```python
from build123d import *

# Parameters (mm, degrees)
SKETCH_R        = 12
SKETCH_R_2      = 1.75
PAD_DEPTH       = 5
PAD001_DEPTH    = 45
PAD002_DEPTH    = 19
POCKET_DEPTH    = 1
SKETCH004_R     = 4.15
POCKET001_DEPTH = 48.001
SKETCH005_R     = 2.6
POCKET002_DEPTH = 42.301
SKETCH006_R     = 2.6
POCKET003_DEPTH = 5
SKETCH008_R     = 1.75
POCKET004_DEPTH = 20.801
SKETCH009_R     = 3.2
POCKET005_DEPTH = 3
POCKET006_DEPTH = 4
SKETCH011_W     = 1
SKETCH011_H     = 8
POCKET007_DEPTH = 18.99
FILLET_R        = 1
FILLET001_R     = 0.5
CHAMFER_SIZE    = 0.49


with BuildPart() as part:
    # Sketch → Pad (new body)
    with BuildSketch(Plane.XY):
        Polygon((0, 0), (-24, 0), (-24, 5), (-15.5, 5), (-15.5, 25), (-24, 25), (-24, 38.3), (-20, 42.3), (26, 42.3), (30, 38.3), (30, 4), (5, -24), (0, -24), align=None)
        with Locations((8.85, 21.15)):
            Circle(SKETCH_R, mode=Mode.SUBTRACT)
        with Locations((-6.65, 36.65)):
            Circle(SKETCH_R_2, mode=Mode.SUBTRACT)
        with Locations((24.35, 36.65)):
            Circle(SKETCH_R_2, mode=Mode.SUBTRACT)
        with Locations((24.35, 5.65)):
            Circle(SKETCH_R_2, mode=Mode.SUBTRACT)
    extrude(amount=PAD_DEPTH)

    # Sketch001 (on Face19 of Pad) → Pad001 (join)
    with BuildSketch(Plane.XY.offset(5)):
        Polygon((0, 0), (-24, 0), (-24, 5), (5, 5), (5, -24), (0, -24), align=None)
    extrude(amount=PAD001_DEPTH)

    # Sketch002 (on Face21 of Pad001) → Pad002 (join)
    with BuildSketch(Plane(origin=(0, 5, 0), x_dir=(-1, 0, 0), z_dir=(0, 1, 0))):
        Polygon((24, 0), (24, 18), (18, 24), (9.2, 24), (3.2, 18), (3.2, 5), (16.5, 5), (16.5, 0), align=None)
    extrude(amount=PAD002_DEPTH)

    # Sketch003 (on Face30 of Pad002) → Pocket (cut)
    with BuildSketch(Plane(origin=(0, 5, 0), x_dir=(-1, 0, 0), z_dir=(0, 1, 0))):
        Polygon((15.5, 0), (15.5, 18), (19.75, 22.25), (24, 18), (24, 0), align=None)
    extrude(amount=POCKET_DEPTH, mode=Mode.SUBTRACT)

    # Sketch004 (on Face37 of Pocket) → Pocket001 (cut, through all)
    with BuildSketch(Plane(origin=(0, 24, 0), x_dir=(-1, 0, 0), z_dir=(0, 1, 0))):
        with Locations((13.6, 15.5)):
            Circle(SKETCH004_R)
    extrude(amount=-POCKET001_DEPTH, mode=Mode.SUBTRACT)

    # Sketch005 (on Face4 of Pocket001) → Pocket002 (cut, through all)
    with BuildSketch(Plane.XZ):
        with Locations((-15, 35)):
            Circle(SKETCH005_R)
    extrude(amount=-POCKET002_DEPTH, mode=Mode.SUBTRACT)

    # Sketch006 (on Face7 of Pocket002) → Pocket003 (cut)
    with BuildSketch(Plane(origin=(0, 0, 0), x_dir=(0, -1, 0), z_dir=(-1, 0, 0))):
        with Locations((15, 40)):
            Circle(SKETCH006_R)
        with Locations((15, 15)):
            Circle(SKETCH006_R)
    extrude(amount=-POCKET003_DEPTH, mode=Mode.SUBTRACT)

    # Sketch008 (on Face41 of Pocket003) → Pocket004 (cut, through all)
    with BuildSketch(Plane.YZ.offset(-3.2)):
        with Locations((15, 8.5)):
            Circle(SKETCH008_R)
    extrude(amount=-POCKET004_DEPTH, mode=Mode.SUBTRACT)

    # Sketch009 (on Face41 of Pocket004) → Pocket005 (cut)
    with BuildSketch(Plane.YZ.offset(-3.2)):
        with Locations((15, 8.5)):
            Circle(SKETCH009_R)
    extrude(amount=-POCKET005_DEPTH, mode=Mode.SUBTRACT)

    # Sketch010 (on Face43 of Pocket005) → Pocket006 (cut)
    with BuildSketch(Plane(origin=(-24, 0, 0), x_dir=(0, -1, 0), z_dir=(-1, 0, 0))):
        Polygon((-12.1, 6.825684), (-12.1, 10.174316), (-15, 11.848632), (-17.9, 10.174316), (-17.9, 6.825684), (-15, 5.151368), align=None)
    extrude(amount=-POCKET006_DEPTH, mode=Mode.SUBTRACT)

    # Sketch011 (on Face36 of Pocket006) → Pocket007 (cut)
    with BuildSketch(Plane(origin=(0, 24, 0), x_dir=(-1, 0, 0), z_dir=(0, 1, 0))):
        with Locations((16, 9)):
            Rectangle(SKETCH011_W, SKETCH011_H)
    extrude(amount=-POCKET007_DEPTH, mode=Mode.SUBTRACT)

    # Fillet
    fillet_edges = [part.edges().sort_by_distance(p)[0] for p in [
        (5, 5, 27.5),
        (-3.2, 24, 11.5),
        (-6.2, 24, 21),
        (-13.6, 24, 24),
        (-21, 24, 21),
        (-24, 24, 9),
        (30, 4, 2.5),
        (-24, 6, 9),
        (-21.875, 6, 20.125),
        (-19.75, 5.5, 22.25),
        (-16.5, 15, 12.531414),
    ]]
    fillet(fillet_edges, radius=FILLET_R)

    # Fillet001
    fillet001_edges = [part.edges().sort_by_distance(p)[0] for p in [
        (-15.5, 15, 11.810488),
    ]]
    fillet(fillet001_edges, radius=FILLET001_R)

    # Chamfer
    chamfer_edges = [part.edges().sort_by_distance(p)[0] for p in [
        (-10.25278, 24, 17.953287),
    ]]
    chamfer(chamfer_edges, length=CHAMFER_SIZE)


solid = part.part
```
Here's how the part is built. I have some questions about the finished solid (model axes, mm). A direction names the side the tool comes from. Coordinates: 2 decimals unless noted, no trailing zeros. Write each loop counter-clockwise with the first axis right and the second up, starting at its lowest first coordinate (ties: lowest second). Pieces come first, ordered by that corner, then holes. Notation, with made-up numbers: (34, -33.75) -> (53, -33.75) arc R21 ccw to (53, -23.75) -> close; hole circle Ø10 at (29.25, 63). An arc over 180 degrees is marked (long way). Use a Markdown table: item, result. Add a question column.
(1) If we section it at C-C, the plane x = 24.35: Write out the boundary of the cut face in (y, z).
(2) If we section it at D-D, the plane x = 7.5: Write out the boundary of the cut face in (y, z).
(3) I'm going to push flat-ended pins straight in: P1, Ø4.5, axis at x = 24.35, y = 36.65, coming from the +Z side; P2, Ø10, axis at x = 9, z = 14.5, coming from the +Y side; P3, Ø5.5, axis at x = -16.5, z = 14.5, coming from the +Y side. Where does each tip first touch, or does it pass through?
(4) We'd pull the mould along Z, two halves only. Please class faces 4 (the flat face through (-17.6, 5.5, 20.1)), 5 (the flat face through (-22.028, 13.57, 5.977)), 6 (the flat face through (-20, 25, 2)), 7 (the flat face through (-6.2, 13.9, 21)): +Z half, -Z half, draft (parallel to the pull), parting line (faces both ways), or undercut.
(5) For faces 1 (the flat face through (-22.03, 16.47, 6)), 2 (the flat face through (0, -12, 25)), 3 (the flat face through (-3.2, 14, 12)), which set-ups out of +Z, -Z, +X, -X, +Y, -Y let a thin tool reach every point of the face, with its end or its side?
(6) Please list where these lines run through material, in increasing order: line 1 (X direction, y = 21, z = 1); line 2 (Z direction, x = 3.5, y = -15); line 3 (Z direction, x = -16, y = 4.5).
(7) If we section it at B-B, the plane y = 36.65: Write out the boundary of the cut face in (x, z).
(8) If we section it at A-A, the plane z = 35: Write out the boundary of the cut face in (x, y).
Outcome:
| question | item | result |
|---|---|---|
| 1 | outline | (-2.33, 0) -> (3.9, 0) -> (3.9, 5) -> (-2.33, 5) -> close; (7.4, 0) -> (34.9, 0) -> (34.9, 5) -> (7.4, 5) -> close; (38.4, 0) -> (42.3, 0) -> (42.3, 5) -> (38.4, 5) -> close |
| 2 | outline | (-21.2, 0) -> (9.23, 0) -> (9.23, 5) -> (-21.2, 5) -> close; (33.07, 0) -> (42.3, 0) -> (42.3, 5) -> (33.07, 5) -> close |
| 3 | P1 | stops at z = 5 |
| 3 | P2 | stops at y = 5 |
| 3 | P3 | stops at y = 24 |
| 4 | face 4 | -Z half |
| 4 | face 5 | undercut |
| 4 | face 6 | draft |
| 4 | face 7 | +Z half |
| 5 | face 1 | -X |
| 5 | face 2 | +Z, -Z, -X, -Y |
| 5 | face 3 | +Z, +X, +Y |
| 6 | line 1 | x = -24 to -16.5, -15.5 to -3.15, 20.85 to 30 |
| 6 | line 2 | z = 0 to 12.4, 17.6 to 37.4, 42.6 to 50 |
| 6 | line 3 | z = 0 to 12.11, 18.89 to 32.6, 37.4 to 50 |
| 7 | outline | (-24, 0) -> (-8.4, 0) -> (-8.4, 5) -> (-24, 5) -> close; (-4.9, 0) -> (22.6, 0) -> (22.6, 5) -> (-4.9, 5) -> close; (26.1, 0) -> (30, 0) -> (30, 5) -> (26.1, 5) -> close |
| 8 | outline | (-24, 0) -> (-17.6, 0) -> (-17.6, 5) -> (-24, 5) -> close; (-12.4, 0) -> (0, 0) -> (0, -24) -> (5, -24) -> (5, 4) arc R1 ccw to (4, 5) -> (-12.4, 5) -> close |
